Model file for the job. Use its own axes, mm. A direction names the side the tool comes from. Give positions to 0.01 mm unless a question says otherwise; leave off trailing zeros. Write each loop counter-clockwise with the first axis right and the second up, starting at its lowest first coordinate (ties: lowest second). Pieces come first, ordered by that corner, then holes.
```python
from build123d import *

# Parameters (mm, degrees)
BASE_FLANGE1_DEPTH          = 102.87
SKETCH6_W                   = 9.525
SKETCH6_H                   = 99.06
CUT_EXTRUDE1_DEPTH          = 10.16
FILLET1_R                   = 21.336
FILLET2_R                   = 12.7
SKETCH8_W                   = 177.8
SKETCH8_H                   = 69.85
CUT_EXTRUDE2_DEPTH          = 10.16
F_27_0_144_DIAMETER_HOLE1_D = 3.6576
F_27_0_144_DIAMETER_HOLE2_D = 3.6576


# Sheet-metal steps are written as plain solids
with BuildPart() as part:
    # Sketch1 → Base-Flange1 (new, symmetric)
    with BuildSketch(Plane.YZ):
        with BuildLine():
            Line((-25.4, -73.66), (-25.4, 15.875))
            ThreePointArc((-25.4, 15.875), (-22.610192091, 22.610192091), (-15.875, 25.4))
            Line((-15.875, 25.4), (171.45, 25.4))
            Line((171.45, 25.4), (171.45, 22.225))
            Line((171.45, 22.225), (-15.875, 22.225))
            ThreePointArc((-15.875, 22.225), (-20.365128061, 20.365128061), (-22.225, 15.875))
            Line((-22.225, 15.875), (-22.225, -73.66))
            Line((-22.225, -73.66), (-25.4, -73.66))
        make_face()
    extrude(amount=BASE_FLANGE1_DEPTH, both=True)

    # Sketch6 → Cut-Extrude1 (cut)
    with BuildSketch(Plane.YZ.offset(102.87)):
        with Locations((-20.6375, -24.13)):
            Rectangle(SKETCH6_W, SKETCH6_H)
    cut_extrude1 = extrude(amount=-CUT_EXTRUDE1_DEPTH, mode=Mode.SUBTRACT)

    # Mirror1: Cut-Extrude1 across plane
    add(cut_extrude1.mirror(Plane(origin=(0, 0, 0), x_dir=(0, 0, 1), z_dir=(1, 0, 0))), mode=Mode.SUBTRACT)

    # Fillet1
    fillet1_edges = [part.edges().sort_by_distance(p)[0] for p in [
        (102.87, 171.45, 23.8125),
        (-102.87, 171.45, 23.8125),
    ]]
    fillet(fillet1_edges, radius=FILLET1_R)

    # Fillet2
    fillet2_edges = [part.edges().sort_by_distance(p)[0] for p in [
        (92.71, -23.8125, -73.66),
        (-92.71, -23.8125, -73.66),
    ]]
    fillet(fillet2_edges, radius=FILLET2_R)

    # Sketch8 → Cut-Extrude2 (cut)
    with BuildSketch(Plane.XY.offset(25.4)):
        with Locations((0, 98.425)):
            Rectangle(SKETCH8_W, SKETCH8_H)
    extrude(amount=-CUT_EXTRUDE2_DEPTH, mode=Mode.SUBTRACT)

    # #27 (0.144) Diameter Hole1 (through all)
    with Locations(Plane.XY.offset(25.4)):
        with Locations((-76.2, 146.05), (-12.7, 146.05), (76.2, 146.05), (76.2, 50.8), (-12.7, 50.8), (-76.2, 50.8)):
            Hole(F_27_0_144_DIAMETER_HOLE1_D / 2)

    # #27 (0.144) Diameter Hole2 (through all)
    with Locations(Plane.XY.offset(25.4)):
        with Locations((92.4814, 160.8074), (95.4278, 92.583), (95.4278, -6.223), (-95.758, 1.016), (-95.758, 85.344), (-92.3544, 160.401), (3.2512, 163.6268)):
            Hole(F_27_0_144_DIAMETER_HOLE2_D / 2)


solid = part.part
```
1. Probe probe 1 along Y at (x, z) = (64, 6) (3 decimals); probe 2 along Z at (x, y) = (-90, 126.5) (3 decimals); probe 3 along Y at (x, z) = (-12, 23). List the from-to ranges inside material, lowest first.
Calculated:
probe 1: y = -25.4 to -22.225
probe 2: z = 22.225 to 25.4
probe 3: y = -22.2 to 49.11, 52.49 to 63.5, 133.35 to 144.36, 147.74 to 171.45
2. Slice it at A-A, the plane x = 42. Write the cut outline in (y, z) (3 decimals).
Calculated:
outline: (-25.4, -73.66) - (-22.225, -73.66) - (-22.225, 15.875) arc R6.35 cw to (-15.875, 22.225) - (63.5, 22.225) - (63.5, 25.4) - (-15.875, 25.4) arc R9.525 ccw to (-25.4, 15.875) - close; (133.35, 22.225) - (171.45, 22.225) - (171.45, 25.4) - (133.35, 25.4) - close
3. Pin check, flat tips, straight feed: P1, Ø4, axis at x = -92.35, y = 160.4, coming from the -Z side (3 decimals); P2, Ø6, axis at x = -24.5, z = -22.5, coming from the +Y side (3 decimals). Stop position of each tip, or through.
Calculated:
P1: stops at z = 22.225
P2: stops at y = -22.225
4. Slice it at B-B, the plane y = 115. Write the cut outline in (x, z) (3 decimals), and give its area (3 significant figures).
Calculated:
outline: (-102.87, 22.225) - (-88.9, 22.225) - (-88.9, 25.4) - (-102.87, 25.4) - close; (88.9, 22.225) - (102.87, 22.225) - (102.87, 25.4) - (88.9, 25.4) - close
area: 88.7 mm2
5. Slice it at C-C, the plane z = -43. Write the cut outline in (x, y) (3 decimals).
Calculated:
outline: (-92.71, -25.4) - (92.71, -25.4) - (92.71, -22.225) - (-92.71, -22.225) - close
6. Which spindle directions (+Z, -Z, +X, -X, +Y, -Y) get a long thin tool onto all of the face, cutting with end or side? Do faces 1 (the flat face through (1, 58, 22.225)), 2 (the cylindrical face through (-89.09, -23.79, -69.84)). Say none if no direction does.
Calculated:
face 1: -Z, +X, -X, +Y
face 2: -Z, -X, +Y, -Y
